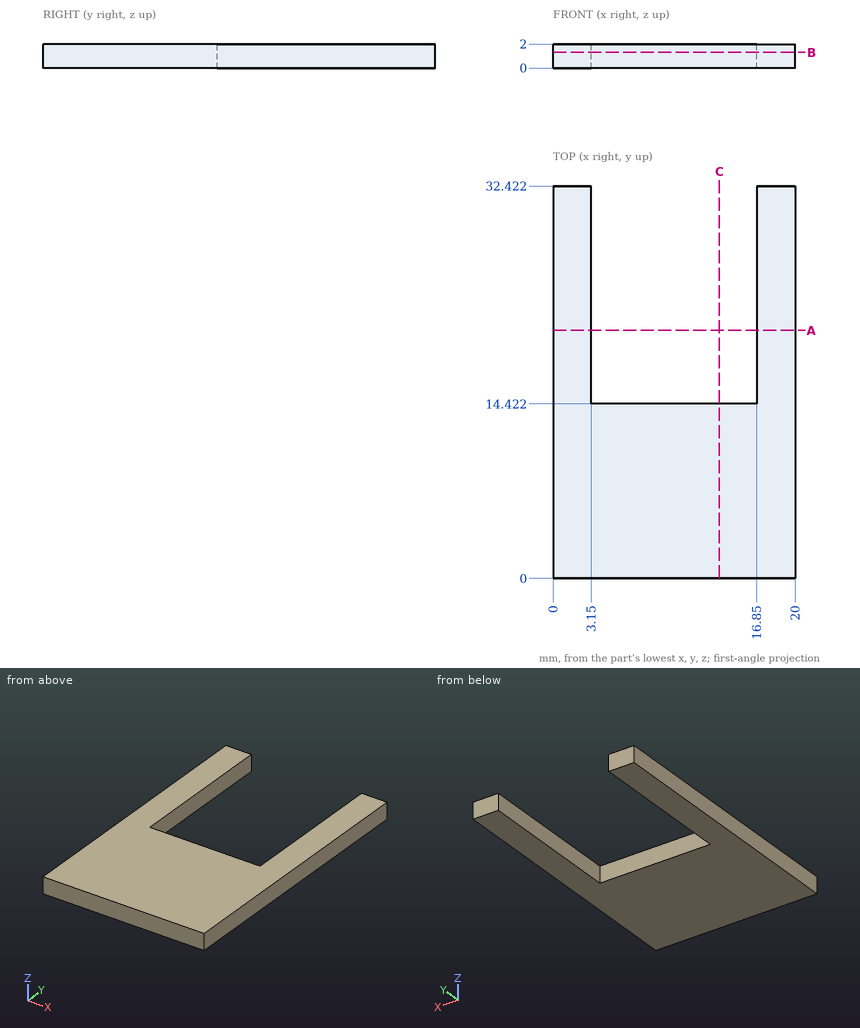
Answer from the drawing. Dimensions are ordinates in mm from the lowest x, y and z of the part. Round coordinates to 2 decimals unless told otherwise and drop trailing zeros. Write each loop counter-clockwise with the first axis right and the second up, starting at its lowest first coordinate (ties: lowest second). Pieces come first, ordered by that corner, then holes.
1. The part is cut by section B-B, the plane z = 1.3. Determine the outline of the cut face in (x, y), then the cut area to 3 significant figures.
2. Given pin 1 Ø12 at (x, y) = (7.5, 15) entering from +Z; pin 2 Ø2 at (x, y) = (13.5, 16.5) entering from -Z; pin 3 Ø1 at (x, z) = (11, 1.5) entering from +Y, each flat-ended and moving along its own axis, determine where each tip first touches the part or whether it passes through.
3. The part is cut by section C-C, the plane x = 13.75. Determine the outline of the cut face in (y, z).
4. Straight lines are drawn through the part: L1, parallel to X at y = 23.5, z = 1.55; L2, parallel to Y at x = 10, z = 0.9. For each, find the intervals that lie inside material, in ascending order.
5. The part is cut by section A-A, the plane y = 20.5. Determine the outline of the cut face in (x, z).
Values:
1. outline: (0, 0) - (20, 0) - (20, 32.42) - (16.85, 32.42) - (16.85, 14.42) - (3.15, 14.42) - (3.15, 32.42) - (0, 32.42) - close
1. area: 402 mm2
2. pin 1: stops at z = 2
2. pin 2: passes through
2. pin 3: stops at y = 14.42
3. outline: (0, 0) - (14.42, 0) - (14.42, 2) - (0, 2) - close
4. L1: x = 0 to 3.15, 16.85 to 20
4. L2: y = 0 to 14.42
5. outline: (0, 0) - (3.15, 0) - (3.15, 2) - (0, 2) - close; (16.85, 0) - (20, 0) - (20, 2) - (16.85, 2) - close
